Autodesk Inventor part; units mm, degrees
ref_plane "YZ Plane" through (0, 0, 0) normal (1, 0, 0) x (0, 1, 0)
ref_plane "XZ Plane" through (0, 0, 0) normal (0, 1, 0) x (-1, 0, 0)
ref_plane "XY Plane" through (0, 0, 0) normal (0, 0, 1) x (1, 0, 0)
sketch "Sketch1" plane through (0, 0, 0) normal (0, 1, 0) x (-1, 0, 0)
  line L0 (93.9879, 313.0349) -> (-256.0121, 313.0349)
  line L1 (-256.0121, 313.0349) -> (-256.0121, -186.9651)
  line L2 (-256.0121, -186.9651) -> (93.9879, -186.9651)
  line L3 (93.9879, -186.9651) -> (93.9879, 313.0349)
  line L4 (27.9879, 283.0349) -> (-190.4121, 283.0349)
  line L5 (-190.4121, 283.0349) -> (-190.4121, 268.0349)
  line L6 (-190.4121, 268.0349) -> (27.9879, 268.0349)
  line L7 (27.9879, 268.0349) -> (27.9879, 283.0349)
  line L8 (27.9879, 217.0349) -> (-190.4121, 217.0349)
  line L9 (-190.4121, 217.0349) -> (-190.4121, 202.0349)
  line L10 (-190.4121, 202.0349) -> (27.9879, 202.0349)
  line L11 (27.9879, 202.0349) -> (27.9879, 217.0349)
  line L12 (27.9879, 151.0349) -> (-190.4121, 151.0349)
  line L13 (-190.4121, 151.0349) -> (-190.4121, 136.0349)
  line L14 (-190.4121, 136.0349) -> (27.9879, 136.0349)
  line L15 (27.9879, 136.0349) -> (27.9879, 151.0349)
  line L16 (27.9879, 85.0349) -> (-190.4121, 85.0349)
  line L17 (-190.4121, 85.0349) -> (-190.4121, 70.0349)
  line L18 (-190.4121, 70.0349) -> (27.9879, 70.0349)
  line L19 (27.9879, 70.0349) -> (27.9879, 85.0349)
  line L20 (27.9879, 19.0349) -> (-190.4121, 19.0349)
  line L21 (-190.4121, 19.0349) -> (-190.4121, 4.0349)
  line L22 (-190.4121, 4.0349) -> (27.9879, 4.0349)
  line L23 (27.9879, 4.0349) -> (27.9879, 19.0349)
  line L24 (27.9879, -46.9651) -> (-190.4121, -46.9651)
  line L25 (-190.4121, -46.9651) -> (-190.4121, -61.9651)
  line L26 (-190.4121, -61.9651) -> (27.9879, -61.9651)
  line L27 (27.9879, -61.9651) -> (27.9879, -46.9651)
  line L28 (27.9879, -112.9651) -> (-190.4121, -112.9651)
  line L29 (-190.4121, -112.9651) -> (-190.4121, -127.9651)
  line L30 (-190.4121, -127.9651) -> (27.9879, -127.9651)
  line L31 (27.9879, -127.9651) -> (27.9879, -112.9651)
  line L32 (27.9879, -186.9651) -> (27.9879, -178.9651)
  line L33 (27.9879, -178.9651) -> (-190.0121, -178.9651)
  line L34 (-190.0121, -178.9651) -> (-190.0121, -186.9651)
  dimension "d0" = 500
  dimension "d1" = 350
  dimension "d11" = 15
  dimension "d13" = 30
  dimension "d22" = 66
  dimension "d27" = 8
  dimension "d28" = 218.4
extrude "Extrusion2" add sketch "Sketch1" against normal blind 8 contours L3 L2 L32 L33 L34 L1 L0 | L2 L34 L33 L32 | L11 L10 L9 L8 | L15 L14 L13 L12 | L19 L18 L17 L16 | L23 L22 L21 L20 | L27 L26 L25 L24 | L31 L30 L29 L28
extrude "Extrusion3" cut sketch "Sketch1" against normal up to surface (8 mm away) contours L11 L10 L9 L8 | L15 L14 L13 L12 | L19 L18 L17 L16 | L23 L22 L21 L20 | L27 L26 L25 L24 | L31 L30 L29 L28
extrude "Extrusion4" cut sketch "Sketch1" against normal up to surface (8 mm away) contours L2 L34 L33 L32
properties part number "ferrite_section" material "Acrylic"
Geometry: final body of the model. Coordinates: model frame, mm. Give positions to 0.01 mm unless a question says otherwise; leave off trailing zeros. Order: outer loops, then holes, each group sorted by start corner. A loop starts at its lowest first (then second) coordinate and runs counter-clockwise, first axis right, second up. Notation, with made-up numbers: (56, 27) - (93, 27) arc R29 ccw to (93, 60) - close; hole circle Ø5 at (78, 8.5). An arc over 180 degrees is marked (long way). Use CSV: the item, a comma, the result in double quotes.
1. Section query B-B (x = 29.5). Give the number of separate pieces and of enclosed holes in the cut face, plus the area to 3 significant figures.
Answers below:
separate pieces,"8"
enclosed holes,"0"
area,"3,100 mm2"
2. Section query A-A (z = -121). Output: boundary loops of the cut face in (x, y).
Answers below:
outline,"(-93.99, -8) - (-27.99, -8) - (-27.99, 0) - (-93.99, 0) - close; (190.41, -8) - (256.01, -8) - (256.01, 0) - (190.41, 0) - close"
3. Contact query for flat-ended pins moving along their axis: pin 1 (2.5 mm diameter, centred on x = 85.5, y = -3.5, fed in from -Z); pin 2 (6 mm diameter, centred on x = 142.5, z = 208, fed in from +Y). Output: stop coordinate, or through.
Answers below:
pin 1,"z = -178.97"
pin 2,"through"
4. Material intervals for line 1 along X through (y, z) = (-1.25, -117), sorted ascending. Write a range as from..to.
Answers below:
line 1,"-93.99..-27.99, 190.41..256.01"
